Could you check a few things on this drawing? It's one solid part, dimensions in mm from its lowest x, y, z. A direction names the side the tool comes from. Give positions to 0.01 mm unless a question says otherwise; leave off trailing zeros. Write each loop counter-clockwise with the first axis right and the second up, starting at its lowest first coordinate (ties: lowest second). Pieces come first, ordered by that corner, then holes. Notation, with made-up numbers: (62, 69.5) -> (83, 69.5) arc R8 ccw to (83, 77.5) -> close; hole circle Ø11 at (58, 34.5). An arc over 180 degrees is marked (long way). Answer as CSV lines item,"result". Start each with the question number.
1. On a 3-axis mill with a long thin cutter (end or side, diameter ignored), from which of +Z, -Z, +X, -X, +Y, -Y can I reach the whole of each face in a straight line? I mean the marked faces 1 and 2. Say none if no direction works.
2. If we section it at A-A on x = 722: Write out the boundary of the cut face in (y, z) (1 decimal).
3. I'm going to push flat-ended pins straight in: P1, Ø12, axis at x = 582, z = 739, coming from the -Y side; P2, Ø6, axis at x = 505.5, z = 600.5, coming from the -Y side (1 decimal); P3, Ø8, axis at x = 594, z = 607.5, coming from the +Y side. Where does each tip first touch, or does it pass through?
4. If we section it at B-B on y = 88.5: Write out the boundary of the cut face in (x, z) (1 decimal).
5. I need wall thicknesses on line 1 (Y direction, x = 326, z = 117.5); line 2 (Y direction, x = 454, z = 504.5); line 3 (X direction, y = 133.5, z = 520) (1 decimal). Which ranges of each line are inside material? Lowest first, please. Write a range as [from, to].
6. If we section it at C-C on y = 31: Write out the boundary of the cut face in (x, z).
7. If we mould it in two halves opening along X, with no side actions, what happens to the marked faces 3, 4 and 5? For each: pulls with the +X half, pulls with the -X half, needs draft (parallel to the pull), parting line crosses it, or undercut.
8. If we section it at D-D on z = 89: Write out the boundary of the cut face in (x, y).
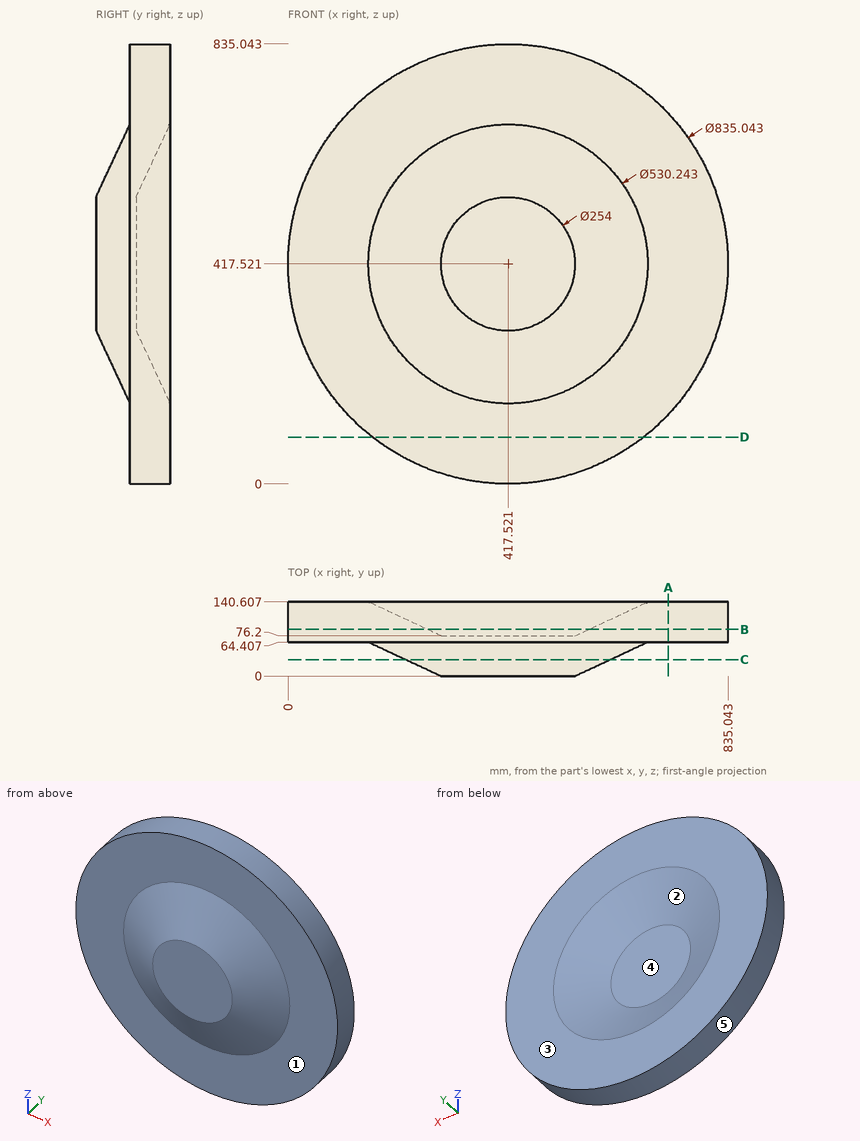
Computed values:
1,face 1,"-Y"
1,face 2,"+Y"
2,outline,"(64.4, 131.8) -> (140.6, 131.8) -> (140.6, 703.2) -> (64.4, 703.2) -> close"
3,P1,"stops at y = 64.41"
3,P2,"stops at y = 34.1"
3,P3,"stops at y = 139.76"
4,outline,"circle Ø835 at (417.5, 417.5); hole circle Ø306.8 at (417.5, 417.5)"
5,line 1,"y = [64.41, 140.61]"
5,line 2,"y = [0, 76.2]"
5,line 3,"x = [12.8, 189.6], [645.4, 822.3]"
6,outline,"circle Ø386.96 at (417.52, 417.52)"
7,face 3,"needs draft"
7,face 4,"undercut"
7,face 5,"parting line crosses it"
8,outline,"(159.84, 64.41) -> (675.2, 64.41) -> (675.2, 140.61) -> (159.84, 140.61) -> close"
